Read the model definition and answer for the solid it produces. Units are mm, in the model's axes. Coordinates: 2 decimals unless noted, no trailing zeros. Order: outer loops, then holes, each group sorted by start corner. A loop starts at its lowest first (then second) coordinate and runs counter-clockwise, first axis right, second up. Notation, with made-up numbers: M 81,-25 L 135,-25 A8 cw 135,-10 Z; hole C -7.5,18 d2. An arc over 180 degrees is marked long. One line per question, with ' | ' between items. Start each with the question number.
1) Find section C-C, the plane z = 12. Write down the section's boundary in (x, y) (1 decimal).
2) Given P1, Ø7, axis at y = 38.1, z = -19.05, coming from the -X side; P2, Ø2, axis at x = -63.5, z = -2.5, coming from the +Y side, each flat-ended and moving along its own axis, determine where each tip first touches the part or whether it passes through.
3) Find section A-A, the plane y = 38.1. Write down the section's boundary in (x, z).
4) Consider probe 1 along Z at (x, y) = (149.35, 38.1); probe 2 along X at (y, z) = (10.5, 10); probe 3 along Y at (x, z) = (-42.5, -18.5) (3 decimals). Determine where each line is inside the solid, lowest interval first.
5) The mould has two halves that part along Y. Classify faces 1 (the face through (149.2, 40.3, 17.4)), 2 (the face through (-4, 0, 1)), 3 (the face through (147.638, 38, -1)): +Y half, -Y half, draft (parallel to the pull), parting line (faces both ways), or undercut.
6) Find section D-D, the plane y = 60. Write down the section's boundary in (x, z), plus the area to 3 significant figures.
from build123d import *

# Parameters (mm, degrees)
F0_W     = 301.625
F0_H     = 88.9
F0_W_2   = 75.00112
F0_H_2   = 75.00112
F1_DEPTH = 3.175
F2_D     = 4.4
F3_W     = 3.175
F3_H     = 88.9
F4_DEPTH = 76.2
F6_D     = 5.5


with BuildPart() as f1:
    # F0 (on Front) → F1 (new body)
    with BuildSketch(Plane.XZ):
        Rectangle(F0_W, F0_H)
        with Locations((-106.35234, 0)):
            Rectangle(F0_W_2, F0_H_2, mode=Mode.SUBTRACT)
        with Locations((-106.35234, 0)):
            Rectangle(F0_W_2, F0_H_2)
    extrude(amount=F1_DEPTH)

    # F2 (through all)
    with Locations(Plane(origin=(0, 0, 0), x_dir=(1, 0, 0), z_dir=(0, 1, 0))):
        with Locations((-143.8529, -37.50056), (-68.85178, -37.50056), (-68.85178, 37.50056), (-143.8529, 37.50056)):
            Hole(F2_D / 2)

    # F3 (on face) → F4 (join)
    with BuildSketch(Plane.XZ):
        with Locations((149.225, 0)):
            Rectangle(F3_W, F3_H)
    extrude(amount=-F4_DEPTH)

    # F6 (through all)
    with Locations(Plane.YZ.offset(150.8125)):
        with Locations((38.1, 19.05), (38.1, -19.05)):
            Hole(F6_D / 2)


solid = f1.part
Report:
1) outline: M -150.8,-3.2 L 150.8,-3.2 L 150.8,76.2 L 147.6,76.2 L 147.6,0 L -150.8,0 Z
2) P1: stops at x = 147.64 | P2: stops at y = 0
3) outline: M 147.64,-44.45 L 150.81,-44.45 L 150.81,-21.8 L 147.64,-21.8 Z; M 147.64,-16.3 L 150.81,-16.3 L 150.81,16.3 L 147.64,16.3 Z; M 147.64,21.8 L 150.81,21.8 L 150.81,44.45 L 147.64,44.45 Z
4) probe 1: z = -44.45 to -21.8, -16.3 to 16.3, 21.8 to 44.45 | probe 2: x = 147.64 to 150.81 | probe 3: y = -3.175 to 0
5) face 1: undercut | face 2: +Y half | face 3: draft
6) outline: M 147.64,-44.45 L 150.81,-44.45 L 150.81,44.45 L 147.64,44.45 Z | area: 282 mm^2
